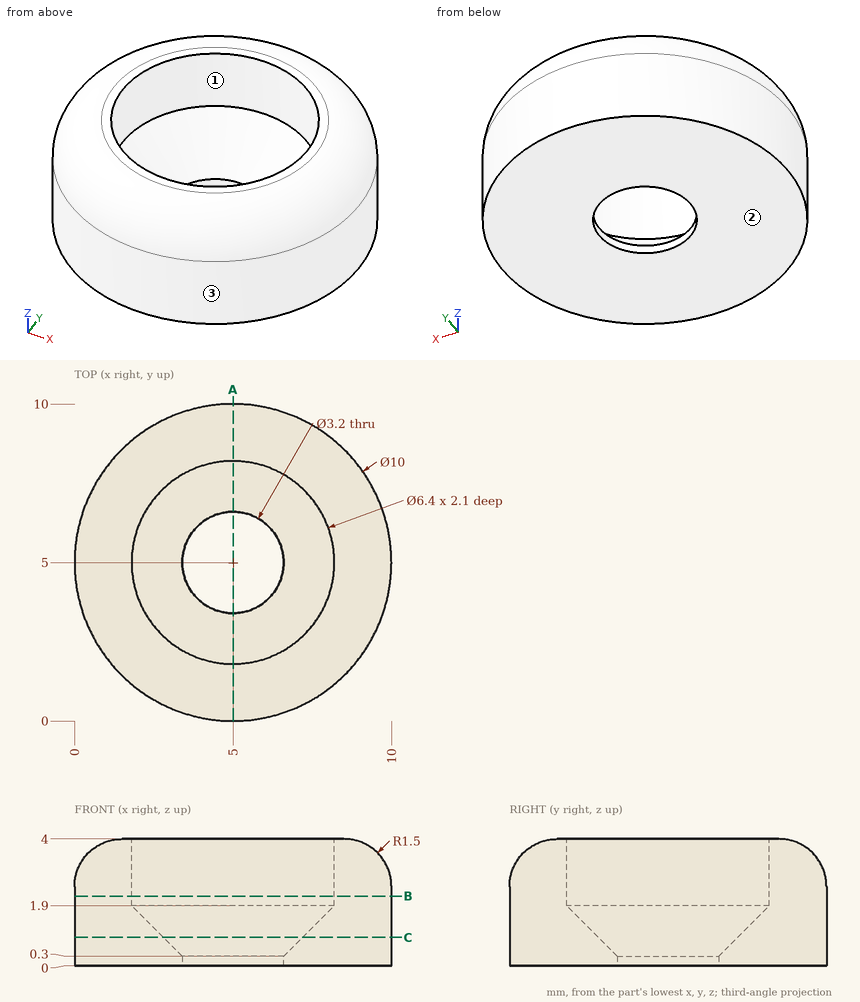
Geometry: see drawing. Coordinates: mm, zero at the bounding-box minimum. Round coordinates to 2 decimals unless told otherwise and drop trailing zeros. Write each loop counter-clockwise with the first axis right and the second up, starting at its lowest first coordinate (ties: lowest second). Pieces come first, ordered by that corner, then holes.
1) Cut plane B-B (z = 2.2). Return the cut outline in (x, y).
2) Cut plane A-A (x = 5). Return the cut outline in (y, z), then the cut area to 3 significant figures.
3) Ray query, L1, parallel to Y at x = 5, z = 0.2; L2, parallel to Y at x = 3.5, z = 3.8; L3, parallel to Z at x = 6.5, y = 8.25. Return the intervals inside material, ascending.
4) Cut plane C-C (z = 0.9). Return the cut outline in (x, y).
5) Draft query along X for the marked faces 1, 2 and 3. Return one class per face: pulls with the +X half, pulls with the -X half, needs draft (parallel to the pull), parting line crosses it, or undercut.
Geometry says:
1. outline: circle Ø10 at (5, 5); hole circle Ø6.4 at (5, 5)
2. outline: (0, 0) - (3.4, 0) - (3.4, 0.3) - (1.8, 1.9) - (1.8, 4) - (1.5, 4) arc R1.5 ccw to (0, 2.5) - close; (6.6, 0) - (10, 0) - (10, 2.5) arc R1.5 ccw to (8.5, 4) - (8.2, 4) - (8.2, 1.9) - (6.6, 0.3) - close
2. area: 17.0 mm2
3. L1: y = 0 to 3.4, 6.6 to 10
3. L2: y = 1.03 to 2.17, 7.83 to 8.97
3. L3: z = 0 to 4
4. outline: circle Ø10 at (5, 5); hole circle Ø4.4 at (5, 5)
5. face 1: undercut
5. face 2: needs draft
5. face 3: parting line crosses it
